from build123d import *

# Parameters (mm, degrees)
SCHIZZO1_W                   = 39
SCHIZZO1_H                   = 15
ESTRUSIONE_ESTRUSIONE1_DEPTH = 2.52
SCHIZZO2_W                   = 39
SCHIZZO2_H                   = 15
SCHIZZO2_W_2                 = 36
SCHIZZO2_H_2                 = 12
TAGLIO_ESTRUSIONE1_DEPTH     = 1
TAGLIO_ESTRUSIONE2_REACH     = 23.044
SCHIZZO3_R                   = 3
ESTRUSIONE_ESTRUSIONE2_START = 1
SCHIZZO4_R                   = 3
ESTRUSIONE_ESTRUSIONE2_DEPTH = 2
SCHIZZO5_W                   = 37
SCHIZZO5_H                   = 13
TAGLIO_ESTRUSIONE4_DEPTH     = 1
TAGLIO_ESTRUSIONE9_DEPTH     = 1.5
ESTRUSIONE_ESTRUSIONE3_START = -1
SCHIZZO11_R                  = 1
ESTRUSIONE_ESTRUSIONE3_DEPTH = 11
SCHIZZO12_R                  = 1
TAGLIO_ESTRUSIONE10_DEPTH    = 1.5
SCHIZZO13_R                  = 4.25
SCHIZZO13_R_2                = 3
ESTRUSIONE_ESTRUSIONE4_DEPTH = 1


with BuildPart() as part:
    # Schizzo1 → Estrusione-Estrusione1 (new body)
    with BuildSketch(Plane.XY):
        Rectangle(SCHIZZO1_W, SCHIZZO1_H)
    extrude(amount=ESTRUSIONE_ESTRUSIONE1_DEPTH)

    # Schizzo2 → Taglio-Estrusione1 (cut)
    with BuildSketch(Plane.XY.offset(2.52)):
        Rectangle(SCHIZZO2_W, SCHIZZO2_H)
        with Locations((-0.5, -0.5)):
            Rectangle(SCHIZZO2_W_2, SCHIZZO2_H_2, mode=Mode.SUBTRACT)
    extrude(amount=-TAGLIO_ESTRUSIONE1_DEPTH, mode=Mode.SUBTRACT)

    # Schizzo3 → Taglio-Estrusione2 (cut, up to next)
    with BuildSketch(Plane.XY.offset(2.52), mode=Mode.PRIVATE) as taglio_estrusione2_sk1:
        with Locations((9, -1)):
            Circle(SCHIZZO3_R)
    taglio_estrusione2_tool1 = extrude(taglio_estrusione2_sk1.sketch, amount=-TAGLIO_ESTRUSIONE2_REACH, mode=Mode.PRIVATE) & part.part
    add(taglio_estrusione2_tool1.solids().sort_by_distance((9, -1, 2.52))[0], mode=Mode.SUBTRACT)

    # Schizzo4 → Estrusione-Estrusione2 (add)
    with BuildSketch(Plane.XY.offset(2.52).offset(ESTRUSIONE_ESTRUSIONE2_START)):
        with BuildLine():
            Line((-0.5, 1.5), (9, 3))
            Line((9, 3), (9, 5.392769143))
            ThreePointArc((9, 5.392769143), (9.117356016, 5.714613176), (9.414334326, 5.885375875))
            ThreePointArc((9.414334326, 5.885375875), (17.276253266, 0.461644492), (12, -7.5))
            Line((12, -7.5), (9.5, -7.5))
            ThreePointArc((9.5, -7.5), (9.146446609, -7.353553391), (9, -7))
            Line((9, -7), (9, -5))
            Line((9, -5), (-0.5, -3.5))
            ThreePointArc((-0.5, -3.5), (-3, -1), (-0.5, 1.5))
        make_face()
        with Locations((9, -1)):
            Circle(SCHIZZO4_R, mode=Mode.SUBTRACT)
        with BuildLine():
            Line((3.448203243, 0.746895178), (2.204268804, 0.186161276))
            ThreePointArc((2.204268804, 0.186161276), (1.959671645, -0.051873187), (1.924787234, -0.391389392))
            ThreePointArc((1.924787234, -0.391389392), (2, -1), (1.924787234, -1.608610608))
            ThreePointArc((1.924787234, -1.608610608), (1.959671645, -1.948126813), (2.204268804, -2.186161276))
            Line((2.204268804, -2.186161276), (3.448203243, -2.746895178))
            ThreePointArc((3.448203243, -2.746895178), (3.972766245, -2.67601261), (4.139708291, -2.173696937))
            ThreePointArc((4.139708291, -2.173696937), (4, -1), (4.139708291, 0.173696937))
            ThreePointArc((4.139708291, 0.173696937), (3.972766245, 0.67601261), (3.448203243, 0.746895178))
        make_face(mode=Mode.SUBTRACT)
    extrude(amount=-ESTRUSIONE_ESTRUSIONE2_DEPTH)

    # Schizzo5 → Taglio-Estrusione4 (cut)
    with BuildSketch(Plane(origin=(0, 0, 0), x_dir=(-1, 0, 0), z_dir=(0, 0, -1))):
        Rectangle(SCHIZZO5_W, SCHIZZO5_H)
    extrude(amount=-TAGLIO_ESTRUSIONE4_DEPTH, mode=Mode.SUBTRACT)

    # Schizzo6 → Taglio-Estrusione9 (cut)
    with BuildSketch(Plane(origin=(0, 0, 0), x_dir=(-1, 0, 0), z_dir=(0, 0, -1))):
        with BuildLine():
            Line((-9, 4.916079783), (-9, 4.153882032))
            ThreePointArc((-9, 4.153882032), (-9.22848325, 3.517673022), (-9.80952381, 3.172190216))
            ThreePointArc((-9.80952381, 3.172190216), (-13.25, -1), (-9.80952381, -5.172190216))
            ThreePointArc((-9.80952381, -5.172190216), (-9.22848325, -5.517673022), (-9, -6.153882032))
            Line((-9, -6.153882032), (-9, -6.916079783))
            ThreePointArc((-9, -6.916079783), (-9.354502776, -7.679842399), (-10.166666667, -7.90209308))
            ThreePointArc((-10.166666667, -7.90209308), (-16, -1), (-10.166666667, 5.90209308))
            ThreePointArc((-10.166666667, 5.90209308), (-9.354502776, 5.679842399), (-9, 4.916079783))
        make_face()
    extrude(amount=-TAGLIO_ESTRUSIONE9_DEPTH, mode=Mode.SUBTRACT)

    # Schizzo11 → Estrusione-Estrusione3 (add)
    with BuildSketch(Plane(origin=(0, 0, 0), x_dir=(-1, 0, 0), z_dir=(0, 0, -1)).offset(ESTRUSIONE_ESTRUSIONE3_START)):
        with Locations(Location((-15.48, -5.864394435, 0), (0, 0, 219.464912598))):
            Circle(SCHIZZO11_R)
        with Locations(Location((-15.48, 6.364394435, 0), (0, 0, 172.206361755))):
            Circle(SCHIZZO11_R)
        with Locations(Location((17.48, 6.364394435, 0), (0, 0, 7.793638245))):
            Circle(SCHIZZO11_R)
        with Locations(Location((17.48, -5.864394435, 0), (0, 0, 219.464912598))):
            Circle(SCHIZZO11_R)
    extrude(amount=ESTRUSIONE_ESTRUSIONE3_DEPTH)

    # Schizzo12 → Taglio-Estrusione10 (cut)
    with BuildSketch(Plane(origin=(0, 0, 1), x_dir=(-1, 0, 0), z_dir=(0, 0, -1))):
        with Locations((-0.2, -2)):
            Circle(SCHIZZO12_R)
    extrude(amount=-TAGLIO_ESTRUSIONE10_DEPTH, mode=Mode.SUBTRACT)

    # Schizzo13 → Estrusione-Estrusione4 (add)
    with BuildSketch(Plane(origin=(0, 0, 1), x_dir=(-1, 0, 0), z_dir=(0, 0, -1))):
        with Locations(Location((-9, -1, 0), (0, 0, 90))):
            Circle(SCHIZZO13_R)
        with Locations(Location((-9, -1, 0), (0, 0, 180))):
            Circle(SCHIZZO13_R_2, mode=Mode.SUBTRACT)
    extrude(amount=ESTRUSIONE_ESTRUSIONE4_DEPTH)


solid = part.part
Design review of the part built by this model. Coordinates are the model's own, in mm. A direction names the side the tool comes from. Give positions to 0.01 mm unless a question says otherwise; leave off trailing zeros. Write each loop counter-clockwise with the first axis right and the second up, starting at its lowest first coordinate (ties: lowest second). Pieces come first, ordered by that corner, then holes. Notation, with made-up numbers: M 40,-28.5 L 91,-28.5 A12 ccw 91,-23.5 Z; hole C 26,73 d8. An arc over 180 degrees is marked long. Answer as a JSON object with one key per item and string values. Group by question number.
1) Tool access review of faces 1 (the face through (3, -1, 2.52)), 2 (the face through (-3, -1, 3)), 3 (the face through (-5, 5.5, 2)), 4 (the face through (17.5, 6.5, 0.5)): name each direction out of +Z, -Z, +X, -X, +Y, -Y from which nothing blocks a thin tool from reaching the whole face with its end or side.
2) We need section B-B (x = 8.5). Give the boundary of the cut face in (y, z), and give its area (3 significant figures).
3) We need section D-D (x = -17.48). Give the boundary of the cut face in (y, z).
4) We need section A-A (x = -7). Give the boundary of the cut face in (y, z), and give its area (3 significant figures).
5) We need section C-C (z = -3). Give the boundary of the cut face in (x, y).
6) Clearance check with flat-ended pins moving along their axes: pin 1 Ø4 at (x, y) = (-10, 0) entering from -Z; pin 2 Ø8 at (y, z) = (-3, -6.5) entering from +X; pin 3 Ø0.8 at (x, z) = (-7, 2) entering from -Y. State where each tip first meets the part, or that it passes through.
7) For line 1 along Y through (x, z) = (0.2, 1.75); line 2 along Z through (x, y) = (-16, 1); line 3 along Y through (x, z) = (15.5, -7.75), list the stretches that pass through material, from the lowest coordinate up.
Answer key:
{
 "1": {"face 1": "+Z", "face 2": "+Z, -X", "face 3": "+Z, -X, +Y", "face 4": "-Z"},
 "2": {"outline": "M -7.5,0 L -6.5,0 L -6.5,1 L -5.22,1 L -5.22,0 L -3.96,0 L -3.96,3.52 L -4.92,3.52 L -4.92,2.52 L -6.5,2.52 L -6.5,1.52 L -7.5,1.52 Z; M 1.96,0 L 3.22,0 L 3.22,1 L 6.5,1 L 6.5,0 L 7.5,0 L 7.5,1.52 L 5.5,1.52 L 5.5,2.52 L 2.92,2.52 L 2.92,3.52 L 1.96,3.52 Z", "area": "17.3 mm²"},
 "3": {"outline": "M -7.5,0 L -6.86,0 L -6.86,-10 L -4.86,-10 L -4.86,1 L 5.36,1 L 5.36,-10 L 7.36,-10 L 7.36,0 L 7.5,0 L 7.5,1.52 L 5.5,1.52 L 5.5,2.52 L -6.5,2.52 L -6.5,1.52 L -7.5,1.52 Z"},
 "4": {"outline": "M -7.5,0 L -6.5,0 L -6.5,1 L 6.5,1 L 6.5,0 L 7.5,0 L 7.5,1.52 L 5.5,1.52 L 5.5,2.52 L -6.5,2.52 L -6.5,1.52 L -7.5,1.52 Z", "area": "21.8 mm²"},
 "5": {"outline": "C -17.48,-5.86 d2; C -17.48,6.36 d2; C 15.48,-5.86 d2; C 15.48,6.36 d2"},
 "6": {"pin 1": "stops at z = 1", "pin 2": "stops at x = 16.48", "pin 3": "stops at y = -6.5"},
 "7": {"line 1": "y = -6.5 to -3, -1 to 5.5", "line 2": "z = 1 to 2.52", "line 3": "y = -6.86 to -4.86, 5.36 to 7.36"}
}
